```python
from build123d import *

# Parameters (mm, degrees)
SKETCH1_R           = 0.6096
BOSS_EXTRUDE1_DEPTH = 1.5875
SKETCH2_W           = 1.5875
SKETCH2_H           = 1.27
BOSS_EXTRUDE2_DEPTH = 2.921
CUT_EXTRUDE1_DEPTH  = 1.5875
SKETCH3_W           = 1.5875
SKETCH3_H           = 5.540367605
CUT_EXTRUDE2_DEPTH  = 1.3335


with BuildPart() as part:
    # Sketch1 → Boss-Extrude1 (new body)
    with BuildSketch(Plane.XY):
        with BuildLine():
            Line((-21.183334762, -18.923), (-7.542517063, -18.923))
            Line((-7.542517063, -18.923), (-1.796769501, -20.710658693))
            Line((-1.796769501, -20.710658693), (-1.796769501, -18.923))
            ThreePointArc((-1.796769501, -18.923), (0, -11.8618), (1.796769501, -18.923))
            Line((1.796769501, -18.923), (1.796769501, -20.710658693))
            Line((1.796769501, -20.710658693), (7.542517063, -18.923))
            Line((7.542517063, -18.923), (21.011390278, -18.923))
            ThreePointArc((21.011390278, -18.923), (24.833026462, -17.340026462), (26.416, -13.518390278))
            Line((26.416, -13.518390278), (26.416, 13.518390278))
            ThreePointArc((26.416, 13.518390278), (24.833026462, 17.340026462), (21.011390278, 18.923))
            Line((21.011390278, 18.923), (-21.183334762, 18.923))
            ThreePointArc((-21.183334762, 18.923), (-24.883387836, 17.390387836), (-26.416, 13.690334762))
            Line((-26.416, 13.690334762), (-26.416, -13.690334762))
            ThreePointArc((-26.416, -13.690334762), (-24.883387836, -17.390387836), (-21.183334762, -18.923))
        make_face()
        with Locations((-22.86, 16.383)):
            Circle(SKETCH1_R, mode=Mode.SUBTRACT)
        with Locations(Location((22.86, 16.383, 0), (0, 0, 180))):
            Circle(SKETCH1_R, mode=Mode.SUBTRACT)
        with Locations((22.86, -16.383)):
            Circle(SKETCH1_R, mode=Mode.SUBTRACT)
        with Locations(Location((-22.86, -16.383, 0), (0, 0, 180))):
            Circle(SKETCH1_R, mode=Mode.SUBTRACT)
        with BuildLine():
            Line((-22.606, 13.690334762), (-22.606, -13.690334762))
            ThreePointArc((-22.606, -13.690334762), (-22.189310999, -14.696310999), (-21.183334762, -15.113))
            Line((-21.183334762, -15.113), (-7.552133781, -15.113))
            Line((-7.552133781, -15.113), (-3.959645297, -10.831638943))
            ThreePointArc((-3.959645297, -10.831638943), (-2.215040295, -9.492956442), (-0.068139526, -9.017))
            Line((-0.068139526, -9.017), (0.068139526, -9.017))
            ThreePointArc((0.068139526, -9.017), (2.215040295, -9.492956442), (3.959645297, -10.831638943))
            Line((3.959645297, -10.831638943), (7.552133781, -15.113))
            Line((7.552133781, -15.113), (21.011390278, -15.113))
            ThreePointArc((21.011390278, -15.113), (22.138949626, -14.645949626), (22.606, -13.518390278))
            Line((22.606, -13.518390278), (22.606, 13.518390278))
            ThreePointArc((22.606, 13.518390278), (22.138949626, 14.645949626), (21.011390278, 15.113))
            Line((21.011390278, 15.113), (-21.183334762, 15.113))
            ThreePointArc((-21.183334762, 15.113), (-22.189310999, 14.696310999), (-22.606, 13.690334762))
        make_face(mode=Mode.SUBTRACT)
    extrude(amount=BOSS_EXTRUDE1_DEPTH)

    # Sketch2 → Boss-Extrude2 (add)
    with BuildSketch(Plane(origin=(-22.606, 0, 0), x_dir=(0, 0, -1), z_dir=(1, 0, 0))):
        with Locations((-0.79375, 3.4798)):
            Rectangle(SKETCH2_W, SKETCH2_H)
        Polygon((0, 1.469264578), (0, 2.8448), (-1.5875, 2.8448), (-1.5875, -6.644691549), (-1.5875, -6.759567605), (0, -6.759567605), align=None)
        Polygon((0, -7.914691549), (0, -6.759567605), (-1.5875, -6.759567605), (-1.5875, -7.914691549), (-1.5875, -8.029567605), (0, -8.029567605), align=None)
    boss_extrude2 = extrude(amount=BOSS_EXTRUDE2_DEPTH)

    # Sketch2<3> → Cut-Extrude1 (cut)
    with BuildSketch(Plane(origin=(-22.606, 0, 0), x_dir=(0, 0, -1), z_dir=(1, 0, 0))):
        Polygon((0, 1.469264578), (0, 2.8448), (-1.5875, 2.8448), (-1.5875, -6.644691549), (-1.5875, -6.759567605), (0, -6.759567605), align=None)
    cut_extrude1 = extrude(amount=CUT_EXTRUDE1_DEPTH, mode=Mode.SUBTRACT)

    # Sketch3 → Cut-Extrude2 (cut)
    with BuildSketch(Plane.ZY.offset(21.0185)):
        with Locations((0.79375, -1.957383802)):
            Rectangle(SKETCH3_W, SKETCH3_H)
    cut_extrude2 = extrude(amount=-CUT_EXTRUDE2_DEPTH, mode=Mode.SUBTRACT)

    # Mirror1: Boss-Extrude2, Cut-Extrude1, Cut-Extrude2 across plane
    add(boss_extrude2.mirror(Plane(origin=(0, 0, 0), x_dir=(0, 0, 1), z_dir=(1, 0, 0))))
    add(cut_extrude1.mirror(Plane(origin=(0, 0, 0), x_dir=(0, 0, 1), z_dir=(1, 0, 0))), mode=Mode.SUBTRACT)
    add(cut_extrude2.mirror(Plane(origin=(0, 0, 0), x_dir=(0, 0, 1), z_dir=(1, 0, 0))), mode=Mode.SUBTRACT)


solid = part.part
```
Can you work these out from the model? Positions are in its coordinate system, mm. Coordinates: 2 decimals unless noted, no trailing zeros. Order: outer loops, then holes, each group sorted by start corner. A loop starts at its lowest first (then second) coordinate and runs counter-clockwise, first axis right, second up.
1. I need wall thicknesses on line 1 (X direction, y = 1.5, z = 1.45) (1 decimal); line 2 (X direction, y = 11, z = 0.5); line 3 (Y direction, x = -22.86, z = 0.75). Which ranges of each line are inside material? Lowest first, please.
2. Thinking about a two-plate mould opening in X: for faces 1 (the face through (-24.924, -17.349, 0.783)), 2 (the face through (-0.4, -9.4, 1.588)), 3 (the face through (21.019, 2, 1)), 4 (the face through (21, 4.115, 1)), which applies, +X half, -X half, draft (parallel to the pull), parting line (faces both ways), or undercut?
3. If we section it at C-C (z = 0.35): Give the number of separate pieces and of enclosed holes in the cut face, then the cut area to 3 significant figures.
4. If we section it at B-B (x = 13): Please give me the cut outline in (y, z).
5. If we section it at A-A (y = 1.5): Please give me the cut outline in (x, z) (1 decimal).
Entries:
1. line 1: x = -26.4 to -22.6, -21 to -19.7, 19.7 to 21, 22.6 to 26.4
1. line 2: x = -26.42 to -22.61, 22.61 to 26.42
1. line 3: y = -18.65 to -16.99, -15.77 to 15.77, 16.99 to 18.65
2. face 1: -X half
2. face 2: draft
2. face 3: undercut
2. face 4: undercut
3. separate pieces: 1
3. enclosed holes: 5
3. area: 658 mm2
4. outline: (-18.92, 0) - (-15.11, 0) - (-15.11, 1.59) - (-18.92, 1.59) - close; (15.11, 0) - (18.92, 0) - (18.92, 1.59) - (15.11, 1.59) - close
5. outline: (-26.4, 0) - (-22.6, 0) - (-22.6, 1.6) - (-26.4, 1.6) - close; (-21, 0) - (-19.7, 0) - (-19.7, 1.6) - (-21, 1.6) - close; (19.7, 0) - (21, 0) - (21, 1.6) - (19.7, 1.6) - close; (22.6, 0) - (26.4, 0) - (26.4, 1.6) - (22.6, 1.6) - close
